```python
from build123d import *

# Parameters (mm, degrees)
BOSS_EXTRUDE1_DEPTH = 1.5
BOSS_EXTRUDE2_DEPTH = 1
SKETCH4_R           = 4.75
CUT_EXTRUDE1_DEPTH  = 23.898325822
SKETCH5_W           = 17.56
SKETCH5_H           = 2.5
BOSS_EXTRUDE3_DEPTH = 0.15
SKETCH6_W           = 17.56
SKETCH6_H           = 2.5
BOSS_EXTRUDE4_DEPTH = 11.35


with BuildPart() as part:
    # Sketch1 → Boss-Extrude1 (new body)
    with BuildSketch(Plane.XY):
        with BuildLine():
            ThreePointArc((14.980604809, 6.55), (8.78, 2), (2.579395191, 6.55))
            Line((2.579395191, 6.55), (0, 6.55))
            Line((0, 6.55), (0, 0))
            Line((0, 0), (17.56, 0))
            Line((17.56, 0), (17.56, 6.55))
            Line((17.56, 6.55), (14.980604809, 6.55))
        make_face()
        with BuildLine():
            ThreePointArc((2.579395191, 6.55), (2.679421093, 10.743420825), (5.32, 14.002581212))
            Line((5.32, 14.002581212), (5.32, 14.619498126))
            ThreePointArc((5.32, 14.619498126), (1.449679407, 11.382680416), (0, 6.55))
            Line((0, 6.55), (2.579395191, 6.55))
        make_face()
        with BuildLine():
            ThreePointArc((12.24, 14.002581212), (14.880578907, 10.743420825), (14.980604809, 6.55))
            Line((14.980604809, 6.55), (17.56, 6.55))
            ThreePointArc((17.56, 6.55), (16.110320593, 11.382680416), (12.24, 14.619498126))
            Line((12.24, 14.619498126), (12.24, 14.002581212))
        make_face()
    extrude(amount=BOSS_EXTRUDE1_DEPTH)

    # Sketch3 → Boss-Extrude2 (add)
    with BuildSketch(Plane.XY.offset(1.5)):
        with BuildLine():
            Line((12.24, 14.619498126), (12.24, 14.002581212))
            ThreePointArc((12.24, 14.002581212), (8.78, 2), (5.32, 14.002581212))
            Line((5.32, 14.002581212), (5.32, 14.619498126))
            ThreePointArc((5.32, 14.619498126), (1.449679407, 11.382680416), (0, 6.55))
            Line((0, 6.55), (0, 0))
            Line((0, 0), (17.56, 0))
            Line((17.56, 0), (17.56, 6.55))
            ThreePointArc((17.56, 6.55), (16.110320593, 11.382680416), (12.24, 14.619498126))
        make_face()
        with BuildLine():
            Line((5.32, 14.619498126), (12.24, 14.619498126))
            Line((12.24, 14.619498126), (12.24, 14.002581212))
            ThreePointArc((12.24, 14.002581212), (8.78, 2), (5.32, 14.002581212))
            Line((5.32, 14.002581212), (5.32, 14.619498126))
        make_face()
    extrude(amount=BOSS_EXTRUDE2_DEPTH)

    # Sketch4 → Cut-Extrude1 (cut, through all)
    with BuildSketch(Plane(origin=(0, 0, 1.5), x_dir=(-1, 0, 0), z_dir=(0, 0, -1))):
        with Locations((-8.78, 8.5)):
            Circle(SKETCH4_R)
    extrude(amount=-CUT_EXTRUDE1_DEPTH, mode=Mode.SUBTRACT)

    # Sketch5 → Boss-Extrude3 (add)
    with BuildSketch(Plane.XZ):
        with Locations((8.78, 1.25)):
            Rectangle(SKETCH5_W, SKETCH5_H)
    extrude(amount=BOSS_EXTRUDE3_DEPTH)

    # Sketch6 → Boss-Extrude4 (add)
    with BuildSketch(Plane.XZ.offset(0.15)):
        with Locations((8.78, 1.25)):
            Rectangle(SKETCH6_W, SKETCH6_H)
    extrude(amount=BOSS_EXTRUDE4_DEPTH)


solid = part.part
```
Input: part model. Units: mm. Frame: model coordinates. Round coordinates to 2 decimals unless told otherwise and drop trailing zeros. Loops run counter-clockwise (first coordinate to the right, second up) from the corner with the lowest first, then second, coordinate; pieces in that order, holes last. Notation, with made-up numbers: (-37, 59.25) -> (8, 59.25) arc R14 ccw to (8, 76.25) -> close; hole circle Ø3 at (-11, 64.25). An arc over 180 degrees is marked (long way). One line per item, written item: value.
(1) Mould query, pull axis X, two halves, no side actions, for faces 1 (the face through (12.55, 5.61, 1.99)), 2 (the face through (12, 13, 1.5)), 3 (the face through (0, -2, 1)), 4 (the face through (9, -1, 2.5)). Classes: pulls with the +X half, pulls with the -X half, needs draft (parallel to the pull), parting line crosses it, or undercut.
Geometry check:
face 1: undercut
face 2: undercut
face 3: pulls with the -X half
face 4: needs draft
(2) Section A-A (x = 8.78). Return the cut outline in (y, z), plus the area to 3 significant figures.
Geometry check:
outline: (-11.5, 0) -> (2, 0) -> (2, 1.5) -> (3.75, 1.5) -> (3.75, 2.5) -> (-11.5, 2.5) -> close; (13.25, 1.5) -> (14.62, 1.5) -> (14.62, 2.5) -> (13.25, 2.5) -> close
area: 36.9 mm2
(3) Section B-B (y = 8.5). Return the cut outline in (x, z).
Geometry check:
outline: (0.22, 0) -> (2.28, 0) -> (2.28, 1.5) -> (4.03, 1.5) -> (4.03, 2.5) -> (0.22, 2.5) -> close; (13.53, 1.5) -> (15.28, 1.5) -> (15.28, 0) -> (17.34, 0) -> (17.34, 2.5) -> (13.53, 2.5) -> close
(4) Section D-D (y = 3). Return the cut outline in (x, z), plus the area to 3 significant figures.
Geometry check:
outline: (0, 0) -> (5.32, 0) -> (5.32, 1.5) -> (12.24, 1.5) -> (12.24, 0) -> (17.56, 0) -> (17.56, 2.5) -> (0, 2.5) -> close
area: 33.5 mm2
(5) Section C-C (z = 1). Return the cut outline in (x, y).
Geometry check:
outline: (0, -11.5) -> (17.56, -11.5) -> (17.56, 6.55) arc R8.78 ccw to (12.24, 14.62) -> (12.24, 14) arc R6.5 cw (long way) to (5.32, 14) -> (5.32, 14.62) arc R8.78 ccw to (0, 6.55) -> close
(6) Material intervals for line 1 (Y direction, x = 8.78, z = 1.7); line 2 (Y direction, x = 11.5, z = 1.6); line 3 (X direction, y = 5.75, z = 2.15), sorted ascending. Write a range as [from, to].
Geometry check:
line 1: [-11.5, 3.75], [13.25, 14.62]
line 2: [-11.5, 4.61], [12.39, 14.62]
line 3: [0, 4.91], [12.65, 17.56]
